```python
from build123d import *

# Parameters (mm, degrees)
SKETCH2_W           = 30
SKETCH2_H           = 19.6
SKETCH2_W_2         = 22
SKETCH2_H_2         = 10
BOSS_EXTRUDE2_DEPTH = 15
SKETCH3_W           = 60
SKETCH3_H           = 60
BOSS_EXTRUDE3_DEPTH = 6.35
FILLET1_R           = 6.35
FILLET2_R           = 2.54
FILLET3_R           = 2.54
FILLET4_R           = 2
SKETCH4_R           = 1.45
CUT_EXTRUDE1_DEPTH  = 45.447300255


with BuildPart() as part:
    # Sketch2 → Boss-Extrude2 (new, symmetric)
    with BuildSketch(Plane(origin=(0, 0, 0), x_dir=(0, 0, -1), z_dir=(1, 0, 0))):
        with Locations((0, -1.55)):
            Rectangle(SKETCH2_W, SKETCH2_H)
        Rectangle(SKETCH2_W_2, SKETCH2_H_2, mode=Mode.SUBTRACT)
    extrude(amount=BOSS_EXTRUDE2_DEPTH, both=True)

    # Sketch3 → Boss-Extrude3 (add)
    with BuildSketch(Plane.XZ.offset(11.35)):
        Rectangle(SKETCH3_W, SKETCH3_H)
    extrude(amount=-BOSS_EXTRUDE3_DEPTH)

    # Fillet1
    fillet1_edges = [part.edges().sort_by_distance(p)[0] for p in [
        (-15, -5, 13),
        (-15, -5, -13),
        (0, -5, 15),
        (15, -5, 13),
        (15, -5, -13),
        (0, -5, -15),
    ]]
    fillet(fillet1_edges, radius=FILLET1_R)

    # Fillet2
    fillet2_edges = [part.edges().sort_by_distance(p)[0] for p in [
        (-15, 8.25, 0),
        (0, 8.25, 15),
        (0, 8.25, -15),
        (15, 8.25, 0),
    ]]
    fillet(fillet2_edges, radius=FILLET2_R)

    # Fillet3
    # the kernel refuses this fillet: 2.54 mm, written as the material it takes off along each edge
    with BuildSketch(Plane(origin=(-15, 5, -11), x_dir=(0, 1, 0), z_dir=(0, 0, 1))) as fillet3_piece_1:
        with BuildLine():
            CenterArc((FILLET3_R, -FILLET3_R), FILLET3_R, 90, 90)
            Line((0, -FILLET3_R), (0, 0))
            Line((0, 0), (FILLET3_R, 0))
        make_face()
    extrude(amount=22, mode=Mode.SUBTRACT)
    with BuildSketch(Plane(origin=(15, 5, -11), x_dir=(0, 1, 0), z_dir=(0, 0, 1))) as fillet3_piece_2:
        with BuildLine():
            CenterArc((FILLET3_R, FILLET3_R), FILLET3_R, 180, 90)
            Line((0, FILLET3_R), (0, 0))
            Line((0, 0), (FILLET3_R, 0))
        make_face()
    extrude(amount=22, mode=Mode.SUBTRACT)

    # Fillet4
    fillet4_edges = [part.edges().sort_by_distance(p)[0] for p in [
        (0, -5, -30),
        (30, -5, 0),
        (0, -5, 30),
        (-30, -5, 0),
    ]]
    fillet(fillet4_edges, radius=FILLET4_R)

    # Sketch4 → Cut-Extrude1 (cut, through all)
    with BuildSketch(Plane(origin=(0, -5, 0), x_dir=(1, 0, 0), z_dir=(0, 1, 0))):
        with Locations(Location((-24.675, 24.675, 0), (0, 0, 270))):
            Circle(SKETCH4_R)
        with Locations(Location((24.675, 24.675, 0), (0, 0, 270))):
            Circle(SKETCH4_R)
        with Locations(Location((24.675, -24.675, 0), (0, 0, 270))):
            Circle(SKETCH4_R)
        with Locations(Location((-24.675, -24.675, 0), (0, 0, 270))):
            Circle(SKETCH4_R)
    extrude(amount=-CUT_EXTRUDE1_DEPTH, mode=Mode.SUBTRACT)


solid = part.part
```
The listing builds one solid part. Answer for the finished solid, in the listing's coordinates (mm). A direction names the side the tool comes from. Coordinates: 2 decimals unless noted, no trailing zeros. Write each loop counter-clockwise with the first axis right and the second up, starting at its lowest first coordinate (ties: lowest second). Pieces come first, ordered by that corner, then holes. Notation, with made-up numbers: (-33, 70) - (-9, 70) arc R16 ccw to (-9, 89) - close; hole circle Ø9 at (-17.5, 54). An arc over 180 degrees is marked (long way). One line per item, written item: value.
1) Each of these flat-tipped pins is pushed along its axis until it touches: pin 1 Ø4.5 at (y, z) = (3, 14) entering from +X; pin 2 Ø4 at (y, z) = (-4, -16.5) entering from +X; pin 3 Ø9.5 at (x, y) = (10, -2) entering from -Z. Where does it stop, or does it pass through?
Geometry check:
pin 1: stops at x = 15.03
pin 2: stops at x = 29.73
pin 3: stops at z = -29.98
2) Find section A-A (x = -11.5). Give the vertices of the cut face in (y, z).
Geometry check:
outline: (-11.35, -30) - (-7, -30) arc R2 ccw to (-5, -28) - (-5, -21.35) arc R6.35 cw to (1.35, -15) - (5.71, -15) arc R2.54 ccw to (8.25, -12.46) - (8.25, 12.46) arc R2.54 ccw to (5.71, 15) - (1.35, 15) arc R6.35 cw to (-5, 21.35) - (-5, 28) arc R2 ccw to (-7, 30) - (-11.35, 30) - close; hole (-5, -11) - (5, -11) - (5, 11) - (-5, 11) - close
3) Find section B-B (z = -9.5). Give the vertices of the cut face in (x, y) (3 decimals), and give its area (3 significant figures).
Geometry check:
outline: (-30, -11.35) - (30, -11.35) - (30, -7) arc R2 ccw to (28, -5) - (-28, -5) arc R2 ccw to (-30, -7) - close; (-14.829, 6.625) arc R2.54 ccw to (-12.46, 5) - (12.46, 5) arc R2.54 ccw to (14.829, 6.625) arc R2.54 ccw to (12.46, 8.25) - (-12.46, 8.25) arc R2.54 ccw to start
area: 471 mm2
4) Consider line 1 along Y through (x, z) = (-12.5, -3); line 2 along Z through (x, y) = (12.5, 3); line 3 along Y through (x, z) = (-18, -6). Determine where each line is inside the solid, lowest interval first. Write a range as from..to.
Geometry check:
line 1: y = -11.35..-5, 5..8.25
line 2: z = -15..-11, 11..15
line 3: y = -11.35..-5
5) For a pull along X with two mould halves and no side action, classify faces 5 (the flat face through (0, -5, 0)), 6 (the flat face through (-30, -9, 0)), 7 (the cylindrical face through (-23.695, -8.131, -25.744)) as pulls with the +X half, pulls with the -X half, needs draft (parallel to the pull), parting line crosses it, or undercut.
Geometry check:
face 5: needs draft
face 6: pulls with the -X half
face 7: undercut
6) A tool of negligible diameter and unlimited length cuts with its end or side. For faces 1 (the flat face through (0, -9, 30)), 2 (the flat face through (15, 4, 13)), 3 (the flat face through (-15, 4, 13)), 4 (the flat face through (0, 5, 0)), from which of +Z, -Z, +X, -X, +Y, -Y can it reach the whole face along a straight path? Write none if from no direction.
Geometry check:
face 1: +Z, +X, -X, +Y, -Y
face 2: +Z, -Z, +X, +Y
face 3: +Z, -Z, -X, +Y
face 4: +X, -X
7) Find section C-C (y = -0.5). Give the vertices of the cut face in (x, z), and give its area (3 significant figures).
Geometry check:
outline: (-15.28, -15.28) - (15.28, -15.28) - (15.28, -11) - (-15.28, -11) - close; (-15.28, 11) - (15.28, 11) - (15.28, 15.28) - (-15.28, 15.28) - close
area: 261 mm2
8) Find section D-D (y = -5.75). Give the vertices of the cut face in (x, z) (3 decimals).
Geometry check:
outline: (-29.561, -29.561) - (29.561, -29.561) - (29.561, 29.561) - (-29.561, 29.561) - close; hole circle Ø2.9 at (-24.675, -24.675); hole circle Ø2.9 at (-24.675, 24.675); hole circle Ø2.9 at (24.675, -24.675); hole circle Ø2.9 at (24.675, 24.675)
